from build123d import *

# Parameters (mm, degrees)
SKETCH1_R           = 76.2
BOSS_EXTRUDE1_DEPTH = 16.256
SHELL1_T            = -3.175
FILLET1_R           = 1.5875
SKETCH2_R           = 38.1
CUT_EXTRUDE1_DEPTH  = 16.256
SKETCH3_R           = 1.524
CUT_EXTRUDE2_DEPTH  = 76.2
CIRPATTERN1_COUNT   = 6
CUT_EXTRUDE4_START  = -1.524
SKETCH5_R           = 76.2
CUT_EXTRUDE4_DEPTH  = 1.524
SKETCH6_R           = 6.35
CUT_EXTRUDE5_DEPTH  = 12.7
SKETCH7_R           = 1.5875
CUT_EXTRUDE6_DEPTH  = 6.35
CUT_EXTRUDE8_DEPTH  = 6.35
CUT_EXTRUDE9_DEPTH  = 6.35


with BuildPart() as part:
    # Sketch1 → Boss-Extrude1 (new body)
    with BuildSketch(Plane(origin=(0, 0, 0), x_dir=(1, 0, 0), z_dir=(0, 1, 0))):
        with Locations(Location((0, 0, 0), (0, 0, 270))):
            Circle(SKETCH1_R)
    extrude(amount=BOSS_EXTRUDE1_DEPTH)

    # Shell1
    shell1_openings = [part.faces().sort_by_distance(p)[0] for p in [
        (0, 16.256, 0),
    ]]
    offset(amount=SHELL1_T, openings=shell1_openings, kind=Kind.INTERSECTION)

    # Fillet1
    fillet1_edges = [part.edges().sort_by_distance(p)[0] for p in [
        (0, 3.175, -73.025),
    ]]
    fillet(fillet1_edges, radius=FILLET1_R)

    # Sketch2 → Cut-Extrude1 (cut)
    with BuildSketch(Plane.XZ):
        with Locations(Location((0, 0, 0), (0, 0, 270))):
            Circle(SKETCH2_R)
    extrude(amount=-CUT_EXTRUDE1_DEPTH, mode=Mode.SUBTRACT)

    # Sketch3 → Cut-Extrude2 (cut)
    with BuildSketch(Plane(origin=(0, 0, 0), x_dir=(0, 0, -1), z_dir=(1, 0, 0))):
        with Locations((0, 8.636)):
            Circle(SKETCH3_R)
    cut_extrude2 = extrude(amount=-CUT_EXTRUDE2_DEPTH, mode=Mode.SUBTRACT)

    # CirPattern1: Cut-Extrude2 ×6 about axis
    cirpattern1_axis = Axis((0, 16.256, 0), (0, -1, 0))
    for i in range(1, CIRPATTERN1_COUNT):
        add(cut_extrude2.rotate(cirpattern1_axis, i * 360 / CIRPATTERN1_COUNT), mode=Mode.SUBTRACT)

    # Sketch5 → Cut-Extrude4 (cut)
    with BuildSketch(Plane(origin=(0, 16.256, 0), x_dir=(1, 0, 0), z_dir=(0, 1, 0)).offset(CUT_EXTRUDE4_START)):
        with Locations(Location((0, 0, 0), (0, 0, 270))):
            Circle(SKETCH5_R)
    extrude(amount=CUT_EXTRUDE4_DEPTH, mode=Mode.SUBTRACT)

    # Sketch6 → Cut-Extrude5 (cut)
    with BuildSketch(Plane(origin=(0, 3.175, 0), x_dir=(1, 0, 0), z_dir=(0, 1, 0))):
        with Locations(Location((0, 64.2874, 0), (0, 0, 270))):
            Circle(SKETCH6_R)
        with Locations(Location((0, -64.2874, 0), (0, 0, 270))):
            Circle(SKETCH6_R)
    extrude(amount=-CUT_EXTRUDE5_DEPTH, mode=Mode.SUBTRACT)

    # Sketch7 → Cut-Extrude6 (cut)
    with BuildSketch(Plane(origin=(0, 3.175, 0), x_dir=(1, 0, 0), z_dir=(0, 1, 0))):
        with Locations(Location((-24.6, 59.525, 0), (0, 0, 270))):
            Circle(SKETCH7_R)
        with Locations(Location((24.6, 59.525, 0), (0, 0, 270))):
            Circle(SKETCH7_R)
        with Locations(Location((24.6, -59.525, 0), (0, 0, 270))):
            Circle(SKETCH7_R)
        with Locations(Location((-24.6, -59.525, 0), (0, 0, 270))):
            Circle(SKETCH7_R)
        with Locations(Location((-59.525, -24.6, 0), (0, 0, 270))):
            Circle(SKETCH7_R)
        with Locations(Location((-59.525, 24.6, 0), (0, 0, 270))):
            Circle(SKETCH7_R)
        with Locations(Location((59.525, 24.6, 0), (0, 0, 270))):
            Circle(SKETCH7_R)
        with Locations(Location((59.525, -24.6, 0), (0, 0, 270))):
            Circle(SKETCH7_R)
    extrude(amount=-CUT_EXTRUDE6_DEPTH, mode=Mode.SUBTRACT)

    # Sketch9 → Cut-Extrude8 (cut)
    with BuildSketch(Plane(origin=(0, 3.175, 0), x_dir=(1, 0, 0), z_dir=(0, 1, 0))):
        with BuildLine():
            Line((-27.700233979, 53.211654386), (-23.272851578, 44.706731925))
            ThreePointArc((-23.272851578, 44.706731925), (-22.741576978, 40.248145008), (-25.292199073, 36.552799702))
            ThreePointArc((-25.292199073, 36.552799702), (-31.430896424, 31.430896424), (-36.552799702, 25.292199073))
            ThreePointArc((-36.552799702, 25.292199073), (-40.248145008, 22.741576978), (-44.706731925, 23.272851578))
            Line((-44.706731925, 23.272851578), (-53.211654386, 27.700233979))
            ThreePointArc((-53.211654386, 27.700233979), (-56.427875079, 31.745110735), (-55.572134976, 36.841463587))
            ThreePointArc((-55.572134976, 36.841463587), (-47.146344636, 47.146344636), (-36.841463587, 55.572134976))
            ThreePointArc((-36.841463587, 55.572134976), (-31.745110735, 56.427875079), (-27.700233979, 53.211654386))
        make_face()
        with BuildLine():
            Line((44.706731925, 23.272851578), (53.211654386, 27.700233979))
            ThreePointArc((53.211654386, 27.700233979), (56.427875079, 31.745110735), (55.572134976, 36.841463587))
            ThreePointArc((55.572134976, 36.841463587), (47.146344636, 47.146344636), (36.841463587, 55.572134976))
            ThreePointArc((36.841463587, 55.572134976), (31.745110735, 56.427875079), (27.700233979, 53.211654386))
            Line((27.700233979, 53.211654386), (23.272851578, 44.706731925))
            ThreePointArc((23.272851578, 44.706731925), (22.741576978, 40.248145008), (25.292199073, 36.552799702))
            ThreePointArc((25.292199073, 36.552799702), (31.430896424, 31.430896424), (36.552799702, 25.292199073))
            ThreePointArc((36.552799702, 25.292199073), (40.248145008, 22.741576978), (44.706731925, 23.272851578))
        make_face()
        with BuildLine():
            Line((27.700233979, -53.211654386), (23.272851578, -44.706731925))
            ThreePointArc((23.272851578, -44.706731925), (22.741576978, -40.248145008), (25.292199073, -36.552799702))
            ThreePointArc((25.292199073, -36.552799702), (31.430896424, -31.430896424), (36.552799702, -25.292199073))
            ThreePointArc((36.552799702, -25.292199073), (40.248145008, -22.741576978), (44.706731925, -23.272851578))
            Line((44.706731925, -23.272851578), (53.211654386, -27.700233979))
            ThreePointArc((53.211654386, -27.700233979), (56.427875079, -31.745110735), (55.572134976, -36.841463587))
            ThreePointArc((55.572134976, -36.841463587), (47.146344636, -47.146344636), (36.841463587, -55.572134976))
            ThreePointArc((36.841463587, -55.572134976), (31.745110735, -56.427875079), (27.700233979, -53.211654386))
        make_face()
        with BuildLine():
            Line((-44.706731925, -23.272851578), (-53.211654386, -27.700233979))
            ThreePointArc((-53.211654386, -27.700233979), (-56.427875079, -31.745110735), (-55.572134976, -36.841463587))
            ThreePointArc((-55.572134976, -36.841463587), (-47.146344636, -47.146344636), (-36.841463587, -55.572134976))
            ThreePointArc((-36.841463587, -55.572134976), (-31.745110735, -56.427875079), (-27.700233979, -53.211654386))
            Line((-27.700233979, -53.211654386), (-23.272851578, -44.706731925))
            ThreePointArc((-23.272851578, -44.706731925), (-22.741576978, -40.248145008), (-25.292199073, -36.552799702))
            ThreePointArc((-25.292199073, -36.552799702), (-31.430896424, -31.430896424), (-36.552799702, -25.292199073))
            ThreePointArc((-36.552799702, -25.292199073), (-40.248145008, -22.741576978), (-44.706731925, -23.272851578))
        make_face()
    extrude(amount=-CUT_EXTRUDE8_DEPTH, mode=Mode.SUBTRACT)

    # Sketch11 → Cut-Extrude9 (cut)
    with BuildSketch(Plane(origin=(0, 3.175, 0), x_dir=(1, 0, 0), z_dir=(0, 1, 0))):
        with BuildLine():
            Line((-48.068824477, 15.156042141), (-57.213344942, 18.039298368))
            ThreePointArc((-57.213344942, 18.039298368), (-62.347716187, 17.453350046), (-65.346282218, 13.244584755))
            ThreePointArc((-65.346282218, 13.244584755), (-66.675, 0), (-65.346282218, -13.244584755))
            ThreePointArc((-65.346282218, -13.244584755), (-62.347716187, -17.453350046), (-57.213344942, -18.039298368))
            Line((-57.213344942, -18.039298368), (-48.068824477, -15.156042141))
            ThreePointArc((-48.068824477, -15.156042141), (-44.540459561, -12.37901297), (-43.731018016, -7.962447065))
            ThreePointArc((-43.731018016, -7.962447065), (-44.45, 0), (-43.731018016, 7.962447065))
            ThreePointArc((-43.731018016, 7.962447065), (-44.540459561, 12.37901297), (-48.068824477, 15.156042141))
        make_face()
        with BuildLine():
            Line((48.068824477, -15.156042141), (57.213344942, -18.039298368))
            ThreePointArc((57.213344942, -18.039298368), (62.347716187, -17.453350046), (65.346282218, -13.244584755))
            ThreePointArc((65.346282218, -13.244584755), (66.675, 0), (65.346282218, 13.244584755))
            ThreePointArc((65.346282218, 13.244584755), (62.347716187, 17.453350046), (57.213344942, 18.039298368))
            Line((57.213344942, 18.039298368), (48.068824477, 15.156042141))
            ThreePointArc((48.068824477, 15.156042141), (44.540459561, 12.37901297), (43.731018016, 7.962447065))
            ThreePointArc((43.731018016, 7.962447065), (44.45, 0), (43.731018016, -7.962447065))
            ThreePointArc((43.731018016, -7.962447065), (44.540459561, -12.37901297), (48.068824477, -15.156042141))
        make_face()
    extrude(amount=-CUT_EXTRUDE9_DEPTH, mode=Mode.SUBTRACT)


solid = part.part
Design review of the part built by this model. Coordinates are the model's own, in mm. A direction names the side the tool comes from. Coordinates: 2 decimals unless noted, no trailing zeros. Order: outer loops, then holes, each group sorted by start corner. A loop starts at its lowest first (then second) coordinate and runs counter-clockwise, first axis right, second up. Notation, with made-up numbers: M 20,46.25 L 66,46.25 A30 cw 66,84.25 Z; hole C 18.5,55.5 d3. An arc over 180 degrees is marked long. Use a Markdown table: item, result.
(1) Draft analysis for pull direction X (two halves, no side actions). For faces 1 (the cylindrical face through (-46.367, 7.263, -60.47)), 2 (the cylindrical face through (5.354, 1.61, 67.701)), 3 (the flat face through (-16, 0, -35)), state which applies: released by +X, released by -X, zero draft, split by the parting line, or undercut.
Worked answers:
| item | result |
|---|---|
| face 1 | split by the parting line |
| face 2 | undercut |
| face 3 | zero draft |
(2) For P1, Ø6, axis at x = -48.5, y = 13, coming from the +Z side; P2, Ø3, axis at y = 8.5, z = -6.5, coming from the +X side; P3, Ø7.5, axis at x = 0, z = 64.29, coming from the +Y side; P4, Ø1.5, axis at x = 39, y = 6, coming from the -Z side, all flat-tipped, find the tip position at first contact; note any pin that passes through.
Worked answers:
| item | result |
|---|---|
| P1 | stops at z = 61.12 |
| P2 | stops at x = 76.04 |
| P3 | passes through |
| P4 | stops at z = -65.9 |
(3) Wall thickness on probe 1 along X at (y, z) = (11, 0) (3 decimals); probe 2 along X at (y, z) = (2, 9.5); probe 3 along Z at (x, y) = (2.5, 9.75): over which ranges is each line inside the solid? List them lowest first.
Worked answers:
| item | result |
|---|---|
| probe 1 | x = -76.2 to -73.025, 73.025 to 76.2 |
| probe 2 | x = -75.61 to -65.99, -43.64 to -36.9, 36.9 to 43.64, 65.99 to 75.61 |
| probe 3 | z = -76.16 to -72.98, 72.98 to 76.16 |
(4) Add section B-B (y = 13). Give the boundary of the cut face in (x, z) (3 decimals).
Worked answers:
| item | result |
|---|---|
| outline | C 0,0 d152.4; hole C 0,0 d146.05 |
(5) Add section A-A (x = 0). Give the boundary of the cut face in (y, z) (1 decimal).
Worked answers:
| item | result |
|---|---|
| outline | M 0,-76.2 L 14.7,-76.2 L 14.7,-73 L 4.8,-73 A1.6 cw 3.2,-71.4 L 3.2,-70.6 L 0,-70.6 Z; M 0,-57.9 L 3.2,-57.9 L 3.2,-38.1 L 0,-38.1 Z; M 0,38.1 L 3.2,38.1 L 3.2,57.9 L 0,57.9 Z; M 0,70.6 L 3.2,70.6 L 3.2,71.4 A1.6 cw 4.8,73 L 14.7,73 L 14.7,76.2 L 0,76.2 Z |
(6) Add section C-C (z = 33.5). Count the separate pieces of the cut face and the enclosed holes in it, then the cut area to 3 significant figures.
Worked answers:
| item | result |
|---|---|
| separate pieces | 4 |
| enclosed holes | 0 |
| area | 229 mm2 |
(7) For faces 4 (the flat face through (-62, 14.732, 39)), 5 (the cylindrical face through (-56.41, 1.61, -31.67)), 6 (the cylindrical face through (21.935, 9.677, 69.653)), list the 3-axis set-ups (+Z, -Z, +X, -X, +Y, -Y) from which the entire face can be reached by the end or side of a thin tool; tool diameter is ignored.
Worked answers:
| item | result |
|---|---|
| face 4 | +Z, -Z, +X, -X, +Y |
| face 5 | +Y, -Y |
| face 6 | +Y |
